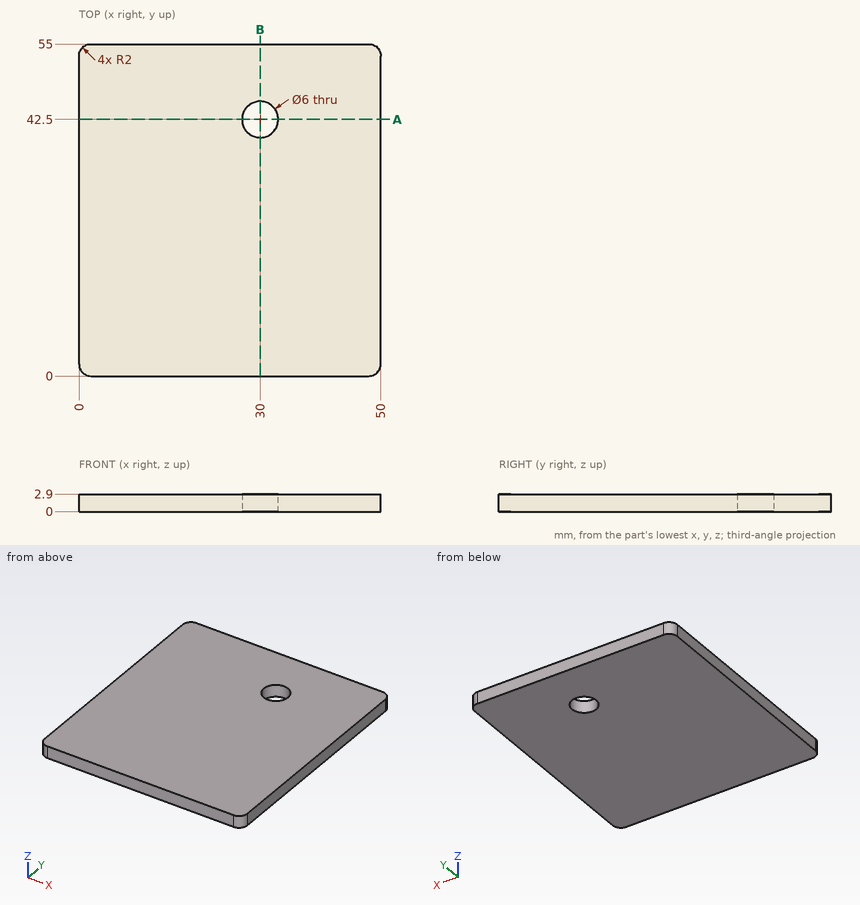
The drawing under review shows one solid part. Ordinate dimensions are in mm from its lowest x, y, z. Round coordinates to 2 decimals unless told otherwise and drop trailing zeros. Write each loop counter-clockwise with the first axis right and the second up, starting at its lowest first coordinate (ties: lowest second). Pieces come first, ordered by that corner, then holes.
(1) Wall thickness on L1, parallel to Y at x = 30, z = 0.75; L2, parallel to X at y = 43, z = 0.9; L3, parallel to X at y = 40, z = 0.2: over which ranges is each line inside the solid? List them lowest first.
(2) Insertion check: pin 1 (3 mm diameter, centred on x = 16.5, y = 49, fed in from -Z); pin 2 (5.5 mm diameter, centred on x = 30, y = 42.5, fed in from +Z). Each pin has a flat end and moves straight along its axis. Give the tip position at first contact, or say it passes through.
(3) We need section B-B on x = 30. Give the boundary of the cut face in (y, z).
(4) We need section A-A on y = 42.5. Give the boundary of the cut face in (x, z), and give its area (3 significant figures).
Findings below:
1. L1: y = 0 to 39.5, 45.5 to 55
1. L2: x = 0 to 27.04, 32.96 to 50
1. L3: x = 0 to 28.34, 31.66 to 50
2. pin 1: stops at z = 0
2. pin 2: passes through
3. outline: (0, 0) - (39.5, 0) - (39.5, 2.9) - (0, 2.9) - close; (45.5, 0) - (55, 0) - (55, 2.9) - (45.5, 2.9) - close
4. outline: (0, 0) - (27, 0) - (27, 2.9) - (0, 2.9) - close; (33, 0) - (50, 0) - (50, 2.9) - (33, 2.9) - close
4. area: 128 mm2
